from build123d import *

# Parameters (mm, degrees)
SKETCH1_W           = 30
SKETCH1_H           = 30
BOSS_EXTRUDE1_DEPTH = 30
FILLET1_R           = 5
FILLET2_R           = 5
FILLET3_R           = 5
FILLET4_R           = 5


with BuildPart() as part:
    # Sketch1 → Boss-Extrude1 (new body)
    with BuildSketch(Plane(origin=(0, 0, 0), x_dir=(1, 0, 0), z_dir=(0, 1, 0))):
        Rectangle(SKETCH1_W, SKETCH1_H)
    extrude(amount=BOSS_EXTRUDE1_DEPTH)

    # Fillet1
    fillet1_edges = [part.edges().sort_by_distance(p)[0] for p in [
        (15, 15, 15),
    ]]
    fillet(fillet1_edges, radius=FILLET1_R)

    # Fillet2
    fillet2_edges = [part.edges().sort_by_distance(p)[0] for p in [
        (15, 15, -15),
    ]]
    fillet(fillet2_edges, radius=FILLET2_R)

    # Fillet3
    fillet3_edges = [part.edges().sort_by_distance(p)[0] for p in [
        (-15, 15, 15),
    ]]
    fillet(fillet3_edges, radius=FILLET3_R)

    # Fillet4
    fillet4_edges = [part.edges().sort_by_distance(p)[0] for p in [
        (-15, 15, -15),
    ]]
    fillet(fillet4_edges, radius=FILLET4_R)


solid = part.part
The listing builds one solid part. Answer for the finished solid, in the listing's coordinates (mm). Coordinates: 2 decimals unless noted, no trailing zeros. Loops run counter-clockwise (first coordinate to the right, second up) from the corner with the lowest first, then second, coordinate; pieces in that order, holes last.
1) Find section B-B on z = 11.75. Write down the section's boundary in (x, y).
2) Find the intervals of material crossed by L1, parallel to X at y = 4.5, z = 10.5; L2, parallel to X at y = 6, z = -11.25; L3, parallel to Z at x = -12.5, y = 2, in increasing order.
3) Find section A-A on y = 5.25. Write down the section's boundary in (x, z), then the cut area to 3 significant figures.
4) Find section C-C on x = -12. Write down the section's boundary in (y, z).
Values:
1. outline: (-14.68, 0) - (14.68, 0) - (14.68, 30) - (-14.68, 30) - close
2. L1: x = -14.97 to 14.97
2. L2: x = -14.84 to 14.84
2. L3: z = -14.33 to 14.33
3. outline: (-15, -10) arc R5 ccw to (-10, -15) - (10, -15) arc R5 ccw to (15, -10) - (15, 10) arc R5 ccw to (10, 15) - (-10, 15) arc R5 ccw to (-15, 10) - close
3. area: 879 mm2
4. outline: (0, -14.58) - (30, -14.58) - (30, 14.58) - (0, 14.58) - close
